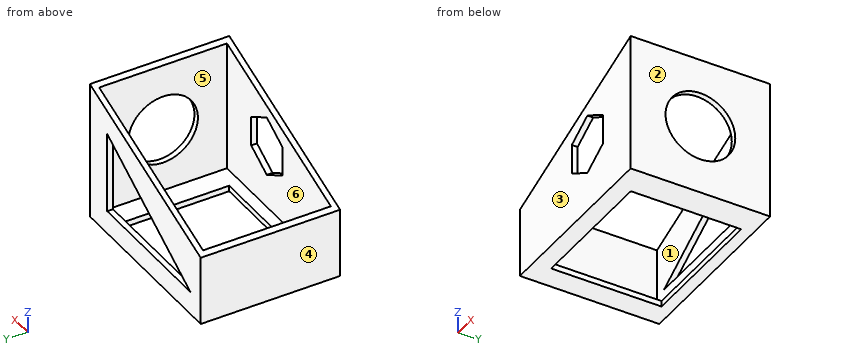
```python
from build123d import *

# Parameters (mm, degrees)
F0_W      = 101.6
F0_H      = 76.2
F1_DEPTH  = 3.175
F2_W      = 101.6
F2_H      = 76.2
F2_W_2    = 95.25
F2_H_2    = 69.85
F3_DEPTH  = 73.025
F5_DEPTH  = 76.201
F6_R      = 19.05
F7_DEPTH  = 25.4
F8_W      = 73.025
F8_H      = 60.325
F9_DEPTH  = 3.176
F11_DEPTH = 25.4
F13_DEPTH = 25.4


with BuildPart() as f1:
    # F0 (on Top) → F1 (new body)
    with BuildSketch(Plane.XY):
        with Locations((2.650434, 1.813662)):
            Rectangle(F0_W, F0_H)
    extrude(amount=F1_DEPTH)

    # F2 (on face) → F3 (join)
    with BuildSketch(Plane.XY.offset(3.175)):
        with Locations((2.650434, 1.813662)):
            Rectangle(F2_W, F2_H)
        with Locations((2.650434, 1.813662)):
            Rectangle(F2_W_2, F2_H_2, mode=Mode.SUBTRACT)
    extrude(amount=F3_DEPTH)

    # F4 (on face) → F5 (cut, through all)
    with BuildSketch(Plane.XZ.offset(36.286338)):
        Polygon((-48.149566, 76.2), (-48.149566, 38.1), (53.450434, 76.2), align=None)
    extrude(amount=-F5_DEPTH, mode=Mode.SUBTRACT)

    # F6 (on face) → F7 (cut)
    with BuildSketch(Plane.YZ.offset(53.450434)):
        with Locations((1.813662, 38.1)):
            Circle(F6_R)
    extrude(amount=-F7_DEPTH, mode=Mode.SUBTRACT)

    # F8 (on face) → F9 (cut, through all)
    with BuildSketch(Plane.XY.offset(3.175)):
        with Locations((1.062934, 3.401162)):
            Rectangle(F8_W, F8_H)
    extrude(amount=-F9_DEPTH, mode=Mode.SUBTRACT)

    # F10 (on face) → F11 (cut)
    with BuildSketch(Plane.XZ.offset(36.286338)):
        Polygon((28.050434, 29.851108), (28.050434, 46.348892), (13.762934, 54.597784), (-0.524566, 46.348892), (-0.524566, 29.851108), (13.762934, 21.602216), align=None)
    extrude(amount=-F11_DEPTH, mode=Mode.SUBTRACT)

    # F12 (on face) → F13 (cut)
    with BuildSketch(Plane(origin=(0, 39.913662, 0), x_dir=(-1, 0, 0), z_dir=(0, 1, 0))):
        Polygon((38.624566, 12.7), (-37.575434, 57.15), (-37.575434, 12.7), align=None)
    extrude(amount=-F13_DEPTH, mode=Mode.SUBTRACT)


solid = f1.part
```
The listing builds one solid part. Answer for the finished solid, in the listing's coordinates (mm). Face numbers are marked on the shaded views. A direction names the side the tool comes from. Round coordinates to 2 decimals unless told otherwise and drop trailing zeros. Loops run counter-clockwise (first coordinate to the right, second up) from the corner with the lowest first, then second, coordinate; pieces in that order, holes last. Notation, with made-up numbers: (-28.5, -6.5) -> (3.5, -6.5) arc R5 ccw to (3.5, 2.5) -> close; hole circle Ø3 at (-6.75, 75.5). An arc over 180 degrees is marked (long way). Use one line per item in the form item = value.
1. Flat-ended cylindrical pins translate along their axes: pin 1 Ø1 at (x, y) = (28, -24.5) entering from +Z; pin 2 Ø23 at (y, z) = (1.81, 38.1) entering from +X; pin 3 Ø1 at (y, z) = (37.5, 38.5) entering from -X; pin 4 Ø1.5 at (x, z) = (2.5, 43.5) entering from -Y. Find the tip coordinate at first contact, or state that the pin passes through.
Answer key:
pin_1 = through
pin_2 = -44.97
pin_3 = -48.15
pin_4 = 36.74
2. The part is cut by section C-C on x = -14. Determine the outline of the cut face in (y, z) (3 decimals).
Answer key:
outline = (-36.286, 0) -> (-26.761, 0) -> (-26.761, 3.175) -> (-33.111, 3.175) -> (-33.111, 50.906) -> (-36.286, 50.906) -> close; (33.564, 0) -> (39.914, 0) -> (39.914, 12.7) -> (36.739, 12.7) -> (36.739, 3.175) -> (33.564, 3.175) -> close; (36.739, 27.064) -> (39.914, 27.064) -> (39.914, 50.906) -> (36.739, 50.906) -> close
3. The part is cut by section B-B on z = 6.5. Determine the outline of the cut face in (x, y), and give its area (3 significant figures).
Answer key:
outline = (-48.15, -36.29) -> (53.45, -36.29) -> (53.45, 39.91) -> (-48.15, 39.91) -> close; hole (-44.97, -33.11) -> (50.28, -33.11) -> (50.28, 36.74) -> (-44.97, 36.74) -> close
area = 1,090 mm²
4. Find the intervals of material crossed by probe 1 along Y at (x, z) = (-28.5, 6.5); probe 2 along Y at (x, z) = (51, 38); probe 3 along X at (y, z) = (-20, 31), in increasing order. Write a range as [from, to].
Answer key:
probe_1 = [-36.29, -33.11], [36.74, 39.91]
probe_2 = [-36.29, -17.24], [20.86, 39.91]
probe_3 = [-48.15, -44.97], [50.28, 53.45]
5. The part is cut by section A-A on y = 31. Determine the outline of the cut face in (x, z) (3 decimals).
Answer key:
outline = (-48.15, 0) -> (-35.45, 0) -> (-35.45, 3.175) -> (-44.975, 3.175) -> (-44.975, 39.291) -> (-48.15, 38.1) -> close; (37.575, 0) -> (53.45, 0) -> (53.45, 76.2) -> (50.275, 75.009) -> (50.275, 3.175) -> (37.575, 3.175) -> close
6. The part is cut by section D-D on y = -7.5. Determine the outline of the cut face in (x, z) (3 decimals), and give its area (3 significant figures).
Answer key:
outline = (-48.15, 0) -> (-35.45, 0) -> (-35.45, 3.175) -> (-44.975, 3.175) -> (-44.975, 39.291) -> (-48.15, 38.1) -> close; (37.575, 0) -> (53.45, 0) -> (53.45, 21.482) -> (50.275, 21.482) -> (50.275, 3.175) -> (37.575, 3.175) -> close; (50.275, 54.718) -> (53.45, 54.718) -> (53.45, 76.2) -> (50.275, 75.009) -> close
area = 328 mm²
7. For a pull along Y with two mould halves and no side action, classify the marked faces 3, 4, 5 and 6 as released by +Y, released by -Y, zero draft, split by the parting line, or undercut.
Answer key:
face_3 = released by -Y
face_4 = zero draft
face_5 = undercut
face_6 = undercut
8. A tool of negligible diameter and unlimited length cuts with its end or side. For the marked faces 1 and 2, from which of +Z, -Z, +X, -X, +Y, -Y can it reach the whole face along a straight path? Write none if from no direction.
Answer key:
face_1 = +Z
face_2 = +Z, -Z, +X, +Y, -Y
